Can you work these out from the drawing? Everything is in mm from the part's minimum corner. A direction names the side the tool comes from. Coordinates: 2 decimals unless noted, no trailing zeros. Order: outer loops, then holes, each group sorted by start corner. A loop starts at its lowest first (then second) coordinate and runs counter-clockwise, first axis right, second up. Notation, with made-up numbers: M 53,5.5 L 104,5.5 A13 cw 104,21.5 Z; hole C -0.75,27.25 d8. An arc over 180 degrees is marked long. Answer as a JSON object with one key per item and string values.
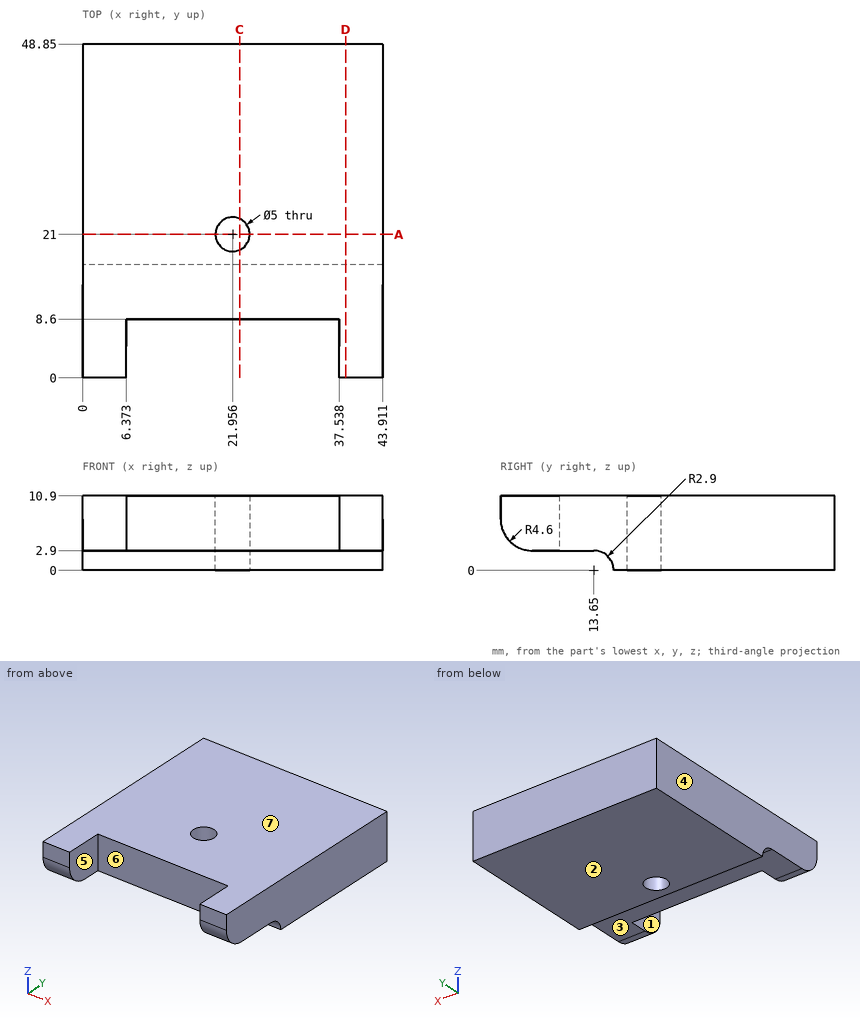
Item 1: I want a section at C-C, the plane x = 23. Write out the boundary of the cut face in (y, z).
Answers follow:
{"outline": "M 8.6,2.9 L 13.65,2.9 A2.9 cw 16.55,0 L 18.73,0 L 18.73,10.9 L 8.6,10.9 Z; M 23.27,0 L 48.85,0 L 48.85,10.9 L 23.27,10.9 Z"}
Item 2: I want a section at D-D, the plane x = 38.5. Write out the boundary of the cut face in (y, z), plus the area to 3 significant figures.
Answers follow:
{"outline": "M 0,7.5 A4.6 ccw 4.6,2.9 L 13.65,2.9 A2.9 cw 16.55,0 L 48.85,0 L 48.85,10.9 L 0,10.9 Z", "area": "482 mm^2"}
Item 3: I want a section at A-A, the plane y = 21. Write out the boundary of the cut face in (x, z) (1 decimal).
Answers follow:
{"outline": "M 0,0 L 19.5,0 L 19.5,10.9 L 0,10.9 Z; M 24.5,0 L 43.9,0 L 43.9,10.9 L 24.5,10.9 Z"}
Item 4: Please list where these lines run through material, in increasing order: line 1 (Y direction, x = 15, z = 5.5); line 2 (Z direction, x = 28.5, y = 12.5); line 3 (X direction, y = 19.5, z = 9) (1 decimal).
Answers follow:
{"line 1": "y = 8.6 to 48.85", "line 2": "z = 2.9 to 10.9", "line 3": "x = 0 to 20, 24 to 43.9"}
Item 5: Which directions (+Z, -Z, +X, -X, +Y, -Y) give clear straight access to the entire face, cutting with the end or side of a thin tool? Please do the marked faces 1, 2 and 3.
Answers follow:
{"face 1": "+Z, -Z, -Y", "face 2": "-Z, +X, -X, +Y, -Y", "face 3": "-Z, +X, -X, -Y"}
Item 6: I'm going to push a flat-ended pin straight in: pin 1 (3 mm diameter, centred on x = 10.5, y = 8.5, fed in from -Z). Where does the tip first touch, or does it pass through?
Answers follow:
{"pin 1": "stops at z = 2.9"}
Item 7: If we mould it in two halves opening along X, with no side actions, what happens to the marked faces 4, 5, 6 and 7? For each: pulls with the +X half, pulls with the -X half, needs draft (parallel to the pull), parting line crosses it, or undercut.
Answers follow:
{"face 4": "pulls with the -X half", "face 5": "undercut", "face 6": "undercut", "face 7": "needs draft"}
